The model under review builds one solid part; all positions refer to its coordinate system, in mm. Face numbers are marked on the shaded views. Give positions to 0.01 mm unless a question says otherwise; leave off trailing zeros. Write each loop counter-clockwise with the first axis right and the second up, starting at its lowest first coordinate (ties: lowest second). Pieces come first, ordered by that corner, then holes. Notation, with made-up numbers: (54.25, 78.5) -> (106.25, 78.5) arc R22 cw to (106.25, 104.5) -> close; hole circle Ø10 at (-5.5, 25.5). An arc over 180 degrees is marked (long way). Use CSV: the item, a comma, the result in double quotes.
```python
from build123d import *

# Parameters (mm, degrees)
ESQUISSE1_W      = 95
ESQUISSE1_H      = 70
EXTRUSION1_DEPTH = 5
ESQUISSE2_W      = 79
ESQUISSE2_H      = 5
ESQUISSE2_W_2    = 58
ESQUISSE2_W_3    = 5
ESQUISSE2_H_2    = 9
EXTRUSION2_DEPTH = 3
ESQUISSE3_W      = 5
ESQUISSE3_H      = 9
EXTRUSION3_DEPTH = 5
CONG_1_R         = 3
ESQUISSE5_R      = 4
ESQUISSE5_R_2    = 1.6
EXTRUSION4_DEPTH = 10
CHANFREIN1_SIZE  = 3
CHANFREIN1_SIZE2 = 8.242432258


with BuildPart() as part:
    # Esquisse1 → Extrusion1 (new body)
    with BuildSketch(Plane(origin=(0, 0, 0), x_dir=(1, 0, 0), z_dir=(0, 1, 0))):
        Rectangle(ESQUISSE1_W, ESQUISSE1_H)
    extrude(amount=EXTRUSION1_DEPTH)

    # Esquisse2 → Extrusion2 (add)
    with BuildSketch(Plane.XZ):
        with Locations((0, 32.5)):
            Rectangle(ESQUISSE2_W, ESQUISSE2_H)
        with Locations((0.5, -32.5)):
            Rectangle(ESQUISSE2_W_2, ESQUISSE2_H)
        with Locations((-45, -10)):
            Rectangle(ESQUISSE2_W_3, ESQUISSE2_H_2)
    extrude(amount=EXTRUSION2_DEPTH)

    # Esquisse3 → Extrusion3 (add)
    with BuildSketch(Plane.XZ):
        with Locations((-45, 5)):
            Rectangle(ESQUISSE3_W, ESQUISSE3_H)
    extrude(amount=EXTRUSION3_DEPTH)

    # Congé1
    cong_1_edges = [part.edges().sort_by_distance(p)[0] for p in [
        (47.5, 2.5, -35),
        (-47.5, 2.5, -35),
        (-47.5, 2.5, 35),
        (47.5, 2.5, 35),
    ]]
    fillet(cong_1_edges, radius=CONG_1_R)

    # Esquisse5 → Extrusion4 (add)
    with BuildSketch(Plane.XZ):
        with Locations((-25.5, 10.5)):
            Circle(ESQUISSE5_R)
        with Locations((-25.5, 10.5)):
            Circle(ESQUISSE5_R_2, mode=Mode.SUBTRACT)
        with Locations((37.3, 9.5)):
            Circle(ESQUISSE5_R)
        with Locations((37.3, 9.5)):
            Circle(ESQUISSE5_R_2, mode=Mode.SUBTRACT)
        with Locations((36.3, -21.9)):
            Circle(ESQUISSE5_R)
        with Locations((36.3, -21.9)):
            Circle(ESQUISSE5_R_2, mode=Mode.SUBTRACT)
        with Locations((-36.5, -23.5)):
            Circle(ESQUISSE5_R)
        with Locations((-36.5, -23.5)):
            Circle(ESQUISSE5_R_2, mode=Mode.SUBTRACT)
    extrude(amount=EXTRUSION4_DEPTH)

    # Chanfrein1
    chanfrein1_edges = [part.edges().sort_by_distance(p)[0] for p in [
        (-29.5, 0, 10.5),
        (32.3, 0, -21.9),
        (-40.5, 0, -23.5),
        (33.3, 0, 9.5),
    ]]
    chanfrein1_side = [part.faces().sort_by_distance(p)[0] for p in [
        (0.586268245, 0, -0.3372194),
    ]]
    chamfer(chanfrein1_edges, length=CHANFREIN1_SIZE, length2=CHANFREIN1_SIZE2, reference=chanfrein1_side[0])


solid = part.part
```
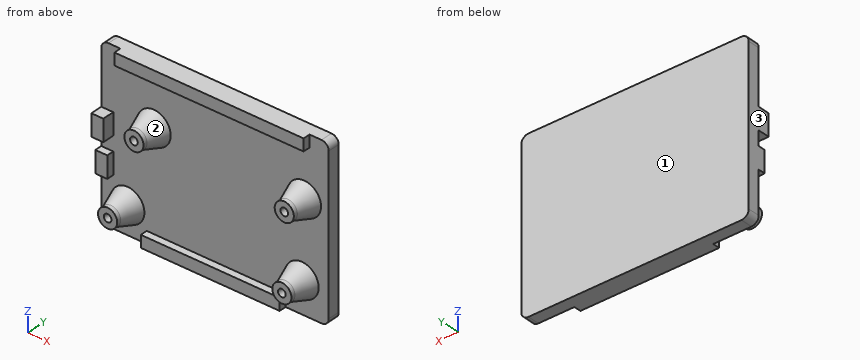
Q1. The part is to be moulded in two halves that separate along X. For the marked faces 1, 2 and 3, say which applies: pulls with the +X half, pulls with the -X half, needs draft (parallel to the pull), parting line crosses it, or undercut.
Derived:
face 1,"needs draft"
face 2,"undercut"
face 3,"pulls with the -X half"
Q2. To check wall thickness, follow probe 1 along Z at (x, y) = (37.3, -4.25); probe 2 along Z at (x, y) = (-2, -1.25); probe 3 along Y at (x, z) = (4.5, 6). State the ranges of each line that lie inside material, in increasing order.
Derived:
probe 1,"z = -27.26 to -23.15, -20.65 to -16.54, 4.05 to 7.9, 11.1 to 14.95"
probe 2,"z = -35 to -30, 30 to 35"
probe 3,"y = 0 to 5"
Q3. Consider section A-A (x = -36.5). Write out the cut boundary in (y, z), then the cut area to 3 significant figures.
Derived:
outline,"(-10, -27.5) -> (-8.24, -27.5) -> (0, -30.5) -> (0, -35) -> (5, -35) -> (5, 35) -> (-3, 35) -> (-3, 30) -> (0, 30) -> (0, -16.5) -> (-8.24, -19.5) -> (-10, -19.5) -> (-10, -21.9) -> (0, -21.9) -> (0, -25.1) -> (-10, -25.1) -> close"
area,"438 mm2"
Q4. Insertion check: pin 1 (2.5 mm diameter, centred on y = -1, z = 33.5, fed in from -X); pin 2 (1.6 mm diameter, centred on x = -36, z = -23.5, fed in from -Y); pin 3 (0.9 mm diameter, centred on x = -44.5, y = -2, fed in from -Z); pin 4 (6 mm diameter, centred on x = -10, y = -7, fed in from -Z). Each pin has a flat end and moves straight along its axis. Give the tip position at first contact, or say it passes through.
Derived:
pin 1,"stops at x = -47.4"
pin 2,"stops at y = 0"
pin 3,"stops at z = -14.5"
pin 4,"passes through"
Q5. Consider section D-D (x = -25.5). Write out the cut boundary in (y, z).
Derived:
outline,"(-10, 6.5) -> (-8.24, 6.5) -> (0, 3.5) -> (0, -30) -> (-3, -30) -> (-3, -35) -> (5, -35) -> (5, 35) -> (-3, 35) -> (-3, 30) -> (0, 30) -> (0, 17.5) -> (-8.24, 14.5) -> (-10, 14.5) -> (-10, 12.1) -> (0, 12.1) -> (0, 8.9) -> (-10, 8.9) -> close"
Q6. Consider section C-C (y = -2). State how many separate pieces and enclosed holes the cut face has, then the cut area to 3 significant figures.
Derived:
separate pieces,"8"
enclosed holes,"4"
area,"1,240 mm2"
Q7. Consider section B-B (y = -7). Write out the cut boundary in (x, z).
Derived:
outline,"circle Ø8.9 at (-36.5, -23.5); circle Ø8.9 at (-25.5, 10.5); circle Ø8.9 at (36.3, -21.9); circle Ø8.9 at (37.3, 9.5); hole circle Ø3.2 at (-36.5, -23.5); hole circle Ø3.2 at (-25.5, 10.5); hole circle Ø3.2 at (36.3, -21.9); hole circle Ø3.2 at (37.3, 9.5)"
